```python
from build123d import *

# Parameters (mm, degrees)
SKETCH1_R           = 1.5
SKETCH1_R_2         = 73
BOSS_EXTRUDE1_DEPTH = 20
SKETCH4_R           = 73
SKETCH4_R_2         = 52.25
BOSS_EXTRUDE2_DEPTH = 10
SKETCH5_R           = 73
BOSS_EXTRUDE3_DEPTH = 10
CUT_EXTRUDE1_DEPTH  = 10
SKETCH7_W           = 155.702807198
SKETCH7_H           = 155.702807198
SKETCH7_R           = 1.5
BOSS_EXTRUDE4_DEPTH = 10
SKETCH8_R           = 1.5
CUT_EXTRUDE2_DEPTH  = 58
SKETCH9_R           = 3
CUT_EXTRUDE3_DEPTH  = 3
SKETCH10_R          = 3
CUT_EXTRUDE4_DEPTH  = 3
SKETCH11_R          = 3
SKETCH11_R_2        = 1.5
BOSS_EXTRUDE6_DEPTH = 3
SKETCH13_R          = 1
CUT_EXTRUDE6_DEPTH  = 5
SKETCH14_R          = 1
CUT_EXTRUDE7_DEPTH  = 5
SKETCH15_R          = 1
CUT_EXTRUDE8_DEPTH  = 5
SKETCH16_R          = 1
CUT_EXTRUDE9_DEPTH  = 5


with BuildPart() as part:
    # Sketch1 → Boss-Extrude1 (new body)
    with BuildSketch(Plane(origin=(0, 0, 0), x_dir=(1, 0, 0), z_dir=(0, 1, 0))):
        with BuildLine():
            Line((77.460838348, -75.098177713), (77.460838348, 74.577424045))
            ThreePointArc((77.460838348, 74.577424045), (76.578174547, 76.708362964), (74.447235628, 77.591026765))
            Line((74.447235628, 77.591026765), (-75.22836613, 77.591026765))
            ThreePointArc((-75.22836613, 77.591026765), (-77.359305049, 76.708362964), (-78.24196885, 74.577424045))
            Line((-78.24196885, 74.577424045), (-78.24196885, -75.098177713))
            ThreePointArc((-78.24196885, -75.098177713), (-77.359305049, -77.229116632), (-75.22836613, -78.111780433))
            Line((-75.22836613, -78.111780433), (74.447235628, -78.111780433))
            ThreePointArc((74.447235628, -78.111780433), (76.578174547, -77.229116632), (77.460838348, -75.098177713))
        make_face()
        with Locations((-60.604326536, -60.47413812)):
            Circle(SKETCH1_R, mode=Mode.SUBTRACT)
        with Locations((-60.604326536, 59.953384452)):
            Circle(SKETCH1_R, mode=Mode.SUBTRACT)
        with Locations((59.823196035, 59.953384452)):
            Circle(SKETCH1_R, mode=Mode.SUBTRACT)
        with Locations((59.823196035, -60.47413812)):
            Circle(SKETCH1_R, mode=Mode.SUBTRACT)
        Circle(SKETCH1_R_2, mode=Mode.SUBTRACT)
    extrude(amount=BOSS_EXTRUDE1_DEPTH)

    # Sketch4 → Boss-Extrude2 (add)
    with BuildSketch(Plane(origin=(0, 20, 0), x_dir=(1, 0, 0), z_dir=(0, 1, 0))):
        Circle(SKETCH4_R)
        Circle(SKETCH4_R_2, mode=Mode.SUBTRACT)
    extrude(amount=-BOSS_EXTRUDE2_DEPTH)

    # Sketch5 → Boss-Extrude3 (add)
    with BuildSketch(Plane.XZ.offset(-10)):
        Circle(SKETCH5_R)
    extrude(amount=BOSS_EXTRUDE3_DEPTH)

    # Sketch6 → Cut-Extrude1 (cut)
    with BuildSketch(Plane(origin=(0, 20, 0), x_dir=(1, 0, 0), z_dir=(0, 1, 0))):
        with BuildLine():
            Line((77.460838348, -75.098177713), (77.460838348, 74.577424045))
            ThreePointArc((77.460838348, 74.577424045), (76.578174547, 76.708362964), (74.447235628, 77.591026765))
            Line((74.447235628, 77.591026765), (-75.22836613, 77.591026765))
            ThreePointArc((-75.22836613, 77.591026765), (-77.359305049, 76.708362964), (-78.24196885, 74.577424045))
            Line((-78.24196885, 74.577424045), (-78.24196885, -75.098177713))
            ThreePointArc((-78.24196885, -75.098177713), (-77.359305049, -77.229116632), (-75.22836613, -78.111780433))
            Line((-75.22836613, -78.111780433), (74.447235628, -78.111780433))
            ThreePointArc((74.447235628, -78.111780433), (76.578174547, -77.229116632), (77.460838348, -75.098177713))
        make_face()
    extrude(amount=-CUT_EXTRUDE1_DEPTH, mode=Mode.SUBTRACT)

    # Sketch7 → Boss-Extrude4 (add)
    with BuildSketch(Plane(origin=(0, 10, 0), x_dir=(1, 0, 0), z_dir=(0, 1, 0))):
        with Locations((-0.390565251, -0.260376834)):
            Rectangle(SKETCH7_W, SKETCH7_H)
        with Locations((59.823196035, 59.953384452)):
            Circle(SKETCH7_R, mode=Mode.SUBTRACT)
        with Locations((59.823196035, -60.47413812)):
            Circle(SKETCH7_R, mode=Mode.SUBTRACT)
        with Locations((-60.604326536, -60.47413812)):
            Circle(SKETCH7_R, mode=Mode.SUBTRACT)
        with Locations((-60.604326536, 59.953384452)):
            Circle(SKETCH7_R, mode=Mode.SUBTRACT)
    extrude(amount=-BOSS_EXTRUDE4_DEPTH)

    # Sketch8 → Cut-Extrude2 (cut)
    with BuildSketch(Plane(origin=(0, 10, 0), x_dir=(1, 0, 0), z_dir=(0, 1, 0))):
        with Locations((-70.24196885, 69.591026765)):
            Circle(SKETCH8_R)
        with Locations((69.460838348, 69.591026765)):
            Circle(SKETCH8_R)
        with Locations((69.460838348, -70.111780433)):
            Circle(SKETCH8_R)
        with Locations((-70.24196885, -70.111780433)):
            Circle(SKETCH8_R)
    extrude(amount=-CUT_EXTRUDE2_DEPTH, mode=Mode.SUBTRACT)

    # Sketch9 → Cut-Extrude3 (cut)
    with BuildSketch(Plane(origin=(0, 10, 0), x_dir=(1, 0, 0), z_dir=(0, 1, 0))):
        with Locations((-60.604326536, 59.953384452)):
            Circle(SKETCH9_R)
        with Locations((59.823196035, 59.953384452)):
            Circle(SKETCH9_R)
        with Locations((59.823196035, -60.47413812)):
            Circle(SKETCH9_R)
        with Locations((-60.604326536, -60.47413812)):
            Circle(SKETCH9_R)
    extrude(amount=-CUT_EXTRUDE3_DEPTH, mode=Mode.SUBTRACT)

    # Sketch10 → Cut-Extrude4 (cut)
    with BuildSketch(Plane.XZ):
        with Locations((59.823196035, -59.953384452)):
            Circle(SKETCH10_R)
        with Locations((-60.604326536, -59.953384452)):
            Circle(SKETCH10_R)
        with Locations((-60.604326536, 60.47413812)):
            Circle(SKETCH10_R)
        with Locations((59.823196035, 60.47413812)):
            Circle(SKETCH10_R)
    extrude(amount=-CUT_EXTRUDE4_DEPTH, mode=Mode.SUBTRACT)

    # Sketch11 → Boss-Extrude6 (add)
    with BuildSketch(Plane(origin=(0, 10, 0), x_dir=(1, 0, 0), z_dir=(0, 1, 0))):
        with Locations((-60.604326536, -60.47413812)):
            Circle(SKETCH11_R)
        with Locations((-60.604326536, -60.47413812)):
            Circle(SKETCH11_R_2, mode=Mode.SUBTRACT)
        with Locations((59.823196035, -60.47413812)):
            Circle(SKETCH11_R)
        with Locations((59.823196035, -60.47413812)):
            Circle(SKETCH11_R_2, mode=Mode.SUBTRACT)
        with Locations((59.823196035, 59.953384452)):
            Circle(SKETCH11_R)
        with Locations((59.823196035, 59.953384452)):
            Circle(SKETCH11_R_2, mode=Mode.SUBTRACT)
        with Locations((-60.604326536, 59.953384452)):
            Circle(SKETCH11_R)
        with Locations((-60.604326536, 59.953384452)):
            Circle(SKETCH11_R_2, mode=Mode.SUBTRACT)
    extrude(amount=-BOSS_EXTRUDE6_DEPTH)

    # Sketch13 → Cut-Extrude6 (cut)
    with BuildSketch(Plane(origin=(0, 0, -77.591026765), x_dir=(-1, 0, 0), z_dir=(0, 0, -1))):
        with Locations((-59.823196035, 5)):
            Circle(SKETCH13_R)
        with Locations((60.604326536, 5)):
            Circle(SKETCH13_R)
    extrude(amount=-CUT_EXTRUDE6_DEPTH, mode=Mode.SUBTRACT)

    # Sketch14 → Cut-Extrude7 (cut)
    with BuildSketch(Plane.ZY.offset(78.24196885)):
        with Locations((-59.953384452, 5)):
            Circle(SKETCH14_R)
        with Locations((60.47413812, 5)):
            Circle(SKETCH14_R)
    extrude(amount=-CUT_EXTRUDE7_DEPTH, mode=Mode.SUBTRACT)

    # Sketch15 → Cut-Extrude8 (cut)
    with BuildSketch(Plane.XY.offset(78.111780433)):
        with Locations((-60.604326536, 5)):
            Circle(SKETCH15_R)
        with Locations((59.823196035, 5)):
            Circle(SKETCH15_R)
    extrude(amount=-CUT_EXTRUDE8_DEPTH, mode=Mode.SUBTRACT)

    # Sketch16 → Cut-Extrude9 (cut)
    with BuildSketch(Plane(origin=(77.460838348, 0, 0), x_dir=(0, 0, -1), z_dir=(1, 0, 0))):
        with Locations((59.953384452, 5)):
            Circle(SKETCH16_R)
        with Locations((-60.47413812, 5)):
            Circle(SKETCH16_R)
    extrude(amount=-CUT_EXTRUDE9_DEPTH, mode=Mode.SUBTRACT)


solid = part.part
```
CAD build for the part. Positions are in the model's coordinates, mm. A direction names the side the tool comes from. Round coordinates to 2 decimals unless told otherwise and drop trailing zeros.
Item 1: Mould opens along Z. For faces 3 (the face through (1, 5, -77.591)), 4 (the face through (61.208, 1.479, 57.813)), 5 (the face through (77.461, 5, 1)) say: pulls with the +Z half, pulls with the -Z half, needs draft (parallel to the pull), parting line crosses it, or undercut.
Item 2: Probe line 1 along Z through (x, y) = (70.5, 4); line 2 along X through (y, z) = (1.5, 58.5). List the from-to ranges inside material, lowest first.
Item 3: Pin check, flat tips, straight feed: pin 1 (0.6 mm diameter, centred on x = 59.5, y = 4.5, fed in from +Z); pin 2 (1.8 mm diameter, centred on y = 5, z = 60.47, fed in from -X); pin 3 (2.5 mm diameter, centred on x = 69.46, z = 70.11, fed in from -Y); pin 4 (1.8 mm diameter, centred on x = -60.6, y = 5, fed in from -Z). Stop position of each tip, or through.
Item 4: Tool access for faces 1 (the face through (62.7, 1.5, -59.1)), 2 (the face through (-1, 0, -1)): list every direction of +Z, -Z, +X, -X, +Y, -Y with a clear straight run to the whole face (end or side of a thin tool).
Reported:
1. face 3: pulls with the -Z half
1. face 4: undercut
1. face 5: needs draft
2. line 1: z = -77.59 to -70.67, -68.51 to 69.03, 71.19 to 78.11
2. line 2: x = -78.24 to -62.86, -58.35 to 57.56, 62.08 to 77.46
3. pin 1: stops at z = 73.11
3. pin 2: stops at x = -73.24
3. pin 3: passes through
3. pin 4: stops at z = -72.59
4. face 1: -Y
4. face 2: +Z, -Z, +X, -X, -Y
